The listing builds one solid part. Answer for the finished solid, in the listing's coordinates (mm). A direction names the side the tool comes from. Coordinates: 2 decimals unless noted, no trailing zeros. Order: outer loops, then holes, each group sorted by start corner. A loop starts at its lowest first (then second) coordinate and runs counter-clockwise, first axis right, second up. Notation, with made-up numbers: (80, -26) -> (115, -26) arc R24 cw to (115, 7) -> close; hole circle Ø1 at (83, 77.25). An arc over 180 degrees is marked (long way). Write item = value, one per line.
from build123d import *

# Parameters (mm, degrees)
SKETCH1_R               = 20
BOSS_EXTRUDE1_DEPTH     = 40
SKETCH2_W               = 10
SKETCH2_H               = 20
CUT_EXTRUDE1_DEPTH      = 40
CUT_EXTRUDE1_DEPTH_BACK = 40
SKETCH3_R               = 10
CUT_EXTRUDE2_DEPTH      = 40
CUT_EXTRUDE2_DEPTH_BACK = 40
CUT_EXTRUDE3_DEPTH      = 10


with BuildPart() as part:
    # Sketch1 → Boss-Extrude1 (new body)
    with BuildSketch(Plane.XY):
        Circle(SKETCH1_R)
    extrude(amount=BOSS_EXTRUDE1_DEPTH)

    # Sketch2 → Cut-Extrude1 (cut, two sides)
    with BuildSketch(Plane(origin=(0, 0, 0), x_dir=(0, 0, -1), z_dir=(1, 0, 0))) as cut_extrude1_sk:
        with Locations((-35, 10)):
            Rectangle(SKETCH2_W, SKETCH2_H)
    extrude(amount=CUT_EXTRUDE1_DEPTH, mode=Mode.SUBTRACT)
    extrude(cut_extrude1_sk.sketch, amount=-CUT_EXTRUDE1_DEPTH_BACK, mode=Mode.SUBTRACT)

    # Sketch3 → Cut-Extrude2 (cut, two sides)
    with BuildSketch(Plane.XY.offset(30)) as cut_extrude2_sk:
        Circle(SKETCH3_R)
    extrude(amount=CUT_EXTRUDE2_DEPTH, mode=Mode.SUBTRACT)
    extrude(cut_extrude2_sk.sketch, amount=-CUT_EXTRUDE2_DEPTH_BACK, mode=Mode.SUBTRACT)

    # Sketch4 → Cut-Extrude3 (cut)
    with BuildSketch(Plane.XY.offset(30)):
        with BuildLine():
            Line((-20, 0), (-10, 0))
            ThreePointArc((-10, 0), (-7.071067812, 7.071067812), (0, 10))
            Line((0, 10), (0, 20))
            ThreePointArc((0, 20), (-14.142135624, 14.142135624), (-20, 0))
        make_face()
    extrude(amount=-CUT_EXTRUDE3_DEPTH, mode=Mode.SUBTRACT)


solid = part.part
Q1. Find the intervals of material crossed by line 1 along Y through (x, z) = (0, 16); line 2 along Z through (x, y) = (13, 2), in increasing order.
The answers:
line_1 = -20 to -10, 10 to 20
line_2 = 0 to 30
Q2. Section D-D, the plane x = 16.5 is taken. Give the vertices of the cut face in (y, z).
The answers:
outline = (-11.3, 0) -> (11.3, 0) -> (11.3, 30) -> (0, 30) -> (0, 40) -> (-11.3, 40) -> close
Q3. Section A-A, the plane x = 7 is taken. Give the vertices of the cut face in (y, z) (3 decimals), plus the area to 3 significant figures.
The answers:
outline = (-18.735, 0) -> (-7.141, 0) -> (-7.141, 40) -> (-18.735, 40) -> close; (7.141, 0) -> (18.735, 0) -> (18.735, 30) -> (7.141, 30) -> close
area = 812 mm2
Q4. Section B-B, the plane z = 3 is taken. Give the vertices of the cut face in (x, y).
The answers:
outline = circle Ø40 at (0, 0); hole circle Ø20 at (0, 0)
Q5. A tool of negligible diameter and unlimited length cuts with its end or side. For faces 1 (the face through (-5, 9, 0)), 2 (the face through (10, 10, 30)), 3 (the face through (-15, 0, 30)), from which of +Z, -Z, +X, -X, +Y, -Y can it reach the whole face along a straight path? Write none if from no direction.
The answers:
face_1 = -Z, +X, -X, +Y, -Y
face_2 = +Z, +X, -X, +Y
face_3 = +Z, -X, +Y
Q6. Section C-C, the plane y = -12 is taken. Give the vertices of the cut face in (x, z).
The answers:
outline = (-16, 0) -> (16, 0) -> (16, 40) -> (-16, 40) -> close
Q7. Each of these flat-tipped pins is pushed along its axis until it touches: pin 1 Ø3 at (y, z) = (13.5, 25.5) entering from -X; pin 2 Ø1.5 at (y, z) = (-16, 20) entering from -X; pin 3 Ø16 at (x, y) = (10.5, 11.5) entering from +Z. Where does it stop, or does it pass through?
The answers:
pin_1 = 0
pin_2 = -12.94
pin_3 = 30
